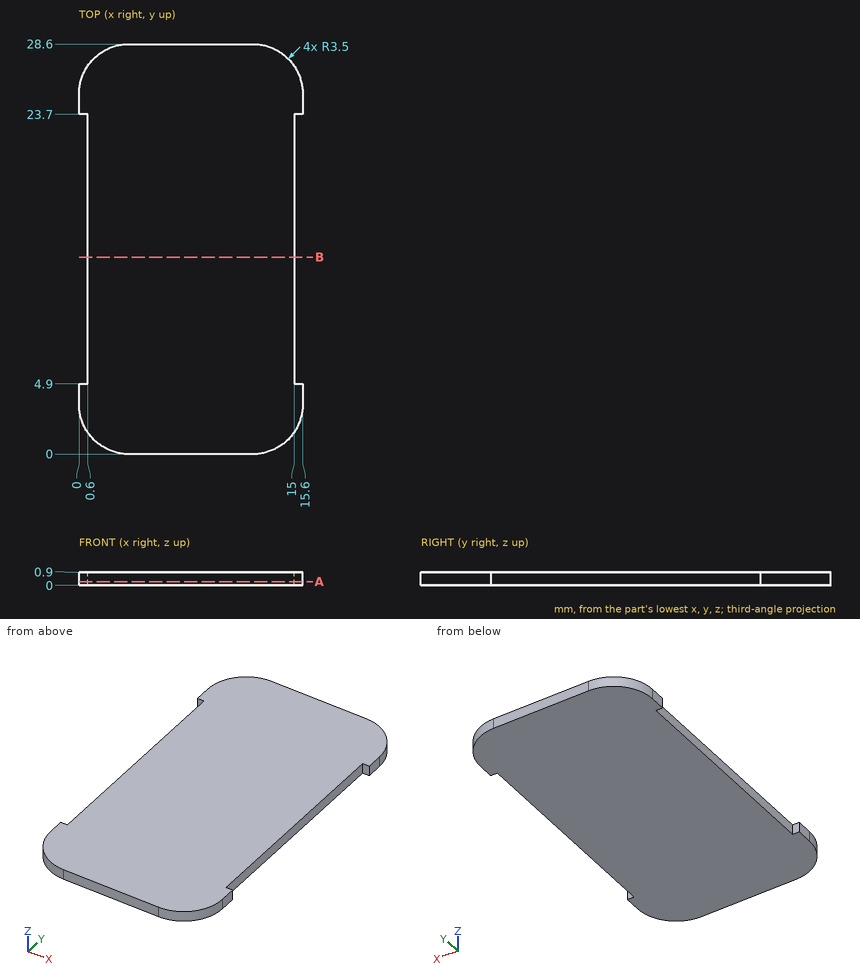
Geometry: see drawing. Coordinates: mm, zero at the bounding-box minimum. Give positions to 0.01 mm unless a question says otherwise; leave off trailing zeros. Loops run counter-clockwise (first coordinate to the right, second up) from the corner with the lowest first, then second, coordinate; pieces in that order, holes last. Notation, with made-up numbers: M 37,86.25 L 67,86.25 A23 ccw 67,94.25 Z; hole C 51,35 d9. An arc over 180 degrees is marked long. Answer as CSV lines item,"result". Start each with the question number.
1. Section A-A on z = 0.25. Return loops of the section in (x, y).
2. Section B-B on y = 13.75. Return loops of the section in (x, z), plus the area to 3 significant figures.
3. Pin query (flat end, axial travel): P1, Ø0.5, axis at x = 0.5, z = 0.5, coming from the +Y side; P2, Ø0.5, axis at y = 17, z = 0.5, coming from the +X side. Return the tip coordinate at first contact, or that it passes through.
4. Line query: L1, parallel to X at y = 6.5, z = 0.7; L2, parallel to Y at x = 12.25, z = 0.55; L3, parallel to Y at x = 14, z = 0.4. Output: solid intervals per line, ascending.
Computed values:
1,outline,"M 0,3.5 A3.5 ccw 3.5,0 L 12.1,0 A3.5 ccw 15.6,3.5 L 15.6,4.9 L 15,4.9 L 15,23.7 L 15.6,23.7 L 15.6,25.1 A3.5 ccw 12.1,28.6 L 3.5,28.6 A3.5 ccw 0,25.1 L 0,23.7 L 0.6,23.7 L 0.6,4.9 L 0,4.9 Z"
2,outline,"M 0.6,0 L 15,0 L 15,0.9 L 0.6,0.9 Z"
2,area,"13.0 mm²"
3,P1,"stops at y = 27.27"
3,P2,"stops at x = 15"
4,L1,"x = 0.6 to 15"
4,L2,"y = 0 to 28.6"
4,L3,"y = 0.56 to 28.04"
